Geometry check sheet. Reference: the model listing, model coordinates, mm. Give positions to 0.01 mm unless a question says otherwise; leave off trailing zeros. Write each loop counter-clockwise with the first axis right and the second up, starting at its lowest first coordinate (ties: lowest second). Pieces come first, ordered by that corner, then holes. Notation, with made-up numbers: (-7.5, 21.5) -> (49.5, 21.5) arc R11 ccw to (49.5, 33.5) -> close; hole circle Ø9 at (29, 48). An arc over 180 degrees is marked (long way). Use a Markdown table: item, result. Add a question column.
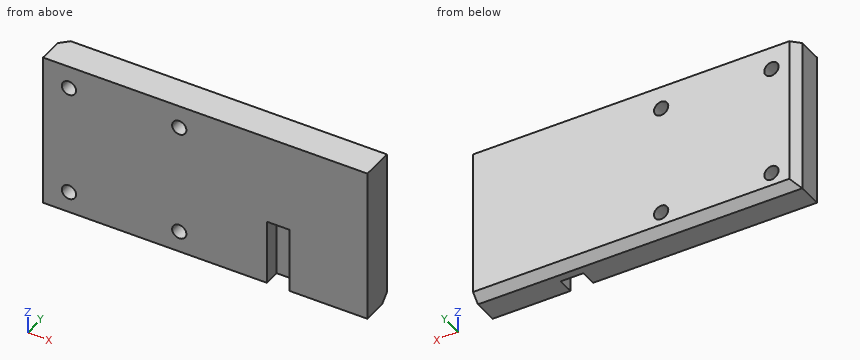
from build123d import *

# Parameters (mm, degrees)
F0_W     = 100
F0_H     = 47.5
F1_DEPTH = 10
F3_D     = 4.4
F2_W     = 7
F2_H     = 20
F4_DEPTH = 5
F5_SIZE  = 2.5


with BuildPart() as f1:
    # F0 (on Front) → F1 (new body)
    with BuildSketch(Plane.XZ):
        with Locations((50, 21.25)):
            Rectangle(F0_W, F0_H)
    extrude(amount=F1_DEPTH)

    # F3 (through all)
    with Locations(Plane.XZ.offset(10)):
        with Locations((8, 38), (42, 38), (42, 4), (8, 4)):
            Hole(F3_D / 2)

    # F2 (on face) → F4 (cut)
    with BuildSketch(Plane.XZ.offset(10)):
        with Locations((72.5, 7.5)):
            Rectangle(F2_W, F2_H)
    extrude(amount=-F4_DEPTH, mode=Mode.SUBTRACT)

    # F5
    f5_edges = [f1.edges().sort_by_distance(p)[0] for p in [
        (0, 0, 21.25),
        (50, 0, -2.5),
    ]]
    chamfer(f5_edges, length=F5_SIZE)


solid = f1.part
1) Sectioned sample at A-A, the plane z = 4. Enter the section's corners in (x, y).
2) Sectioned sample at B-B, the plane x = 42. Enter the section's corners in (y, z).
3) Material ranges on probe 1 along Z at (x, y) = (8, -2.5); probe 2 along X at (y, z) = (-9.5, 17); probe 3 along X at (y, z) = (-3.5, 39), recorded low to high. Write a range as [from, to].
4) Sectioned sample at D-D, the plane z = 38. Enter the section's corners in (x, y).
5) Gauge pin test, flat end, axial feed: P1, Ø2.5, axis at x = 73, y = -8.5, coming from the -Z side. Record the tip position at first contact, or that the pin passes through.
6) Sectioned sample at C-C, the plane z = 16.5. Enter the section's corners in (x, y), and give its area (3 significant figures).
Check values:
| question | item | result |
|---|---|---|
| 1 | outline | (0, -10) -> (5.8, -10) -> (5.8, 0) -> (2.5, 0) -> (0, -2.5) -> close; (10.2, -10) -> (39.8, -10) -> (39.8, 0) -> (10.2, 0) -> close; (44.2, -10) -> (69, -10) -> (69, -5) -> (76, -5) -> (76, -10) -> (100, -10) -> (100, 0) -> (44.2, 0) -> close |
| 2 | outline | (-10, -2.5) -> (-2.5, -2.5) -> (0, 0) -> (0, 1.8) -> (-10, 1.8) -> close; (-10, 6.2) -> (0, 6.2) -> (0, 35.8) -> (-10, 35.8) -> close; (-10, 40.2) -> (0, 40.2) -> (0, 45) -> (-10, 45) -> close |
| 3 | probe 1 | [-2.5, 1.8], [6.2, 35.8], [40.2, 45] |
| 3 | probe 2 | [0, 69], [76, 100] |
| 3 | probe 3 | [0, 6.04], [9.96, 40.04], [43.96, 100] |
| 4 | outline | (0, -10) -> (5.8, -10) -> (5.8, 0) -> (2.5, 0) -> (0, -2.5) -> close; (10.2, -10) -> (39.8, -10) -> (39.8, 0) -> (10.2, 0) -> close; (44.2, -10) -> (100, -10) -> (100, 0) -> (44.2, 0) -> close |
| 5 | P1 | z = 17.5 |
| 6 | outline | (0, -10) -> (69, -10) -> (69, -5) -> (76, -5) -> (76, -10) -> (100, -10) -> (100, 0) -> (2.5, 0) -> (0, -2.5) -> close |
| 6 | area | 962 mm² |
